The listing builds one solid part. Answer for the finished solid, in the listing's coordinates (mm). A direction names the side the tool comes from. Coordinates: 2 decimals unless noted, no trailing zeros. Loops run counter-clockwise (first coordinate to the right, second up) from the corner with the lowest first, then second, coordinate; pieces in that order, holes last. Notation, with made-up numbers: (68.5, -6.5) -> (89.5, -6.5) arc R25 cw to (89.5, 19.5) -> close; hole circle Ø1 at (70, -30.75). An arc over 180 degrees is marked (long way). Answer in a Markdown table with one row per item.
```python
from build123d import *

# Parameters (mm, degrees)
PAD003_DEPTH        = 1.6
SKETCH006_R         = 3.75
PAD004_DEPTH        = 3.6
HOLE001_D           = 3.6
HOLE001_DEPTH       = 25
HOLE001_CSINK_D     = 6.7
HOLE001_CSINK_ANGLE = 90


with BuildPart() as part:
    # Sketch005 → Pad003 (new body)
    with BuildSketch(Plane.XY):
        with BuildLine():
            Line((-49.75, 4.75), (49.75, 4.75))
            ThreePointArc((49.75, -4.75), (54.5, 0), (49.75, 4.75))
            Line((49.75, -4.75), (-49.75, -4.75))
            ThreePointArc((-49.75, 4.75), (-54.5, 0), (-49.75, -4.75))
        make_face()
    extrude(amount=PAD003_DEPTH)

    # Sketch006 → Pad004 (join)
    with BuildSketch(Plane.XY):
        with Locations((-49.75, 0)):
            Circle(SKETCH006_R)
        with Locations((-9.75, 0)):
            Circle(SKETCH006_R)
        with Locations((9.75, 0)):
            Circle(SKETCH006_R)
        with Locations((49.75, 0)):
            Circle(SKETCH006_R)
    extrude(amount=PAD004_DEPTH)

    # Hole001
    with Locations(Plane(origin=(0, 0, 0), x_dir=(1, 0, 0), z_dir=(0, 0, -1))):
        with Locations((-49.75, 0), (-9.75, 0), (9.75, 0), (49.75, 0)):
            CounterSinkHole(HOLE001_D / 2, HOLE001_CSINK_D / 2, depth=HOLE001_DEPTH, counter_sink_angle=HOLE001_CSINK_ANGLE)


with BuildPart() as part_1:
    # Body001 placement: moved
    add(part.part.moved(Location((0, 36, -32))))


solid = part_1.part
```
Item 1: A cutting plane is placed at C-C, the plane y = 36. Count the separate pieces of the cut face and the enclosed holes in it, plus the area to 3 significant figures.
Findings below:
| item | result |
|---|---|
| separate pieces | 5 |
| enclosed holes | 0 |
| area | 173 mm2 |
Item 2: A cutting plane is placed at A-A, the plane z = -29.75. Determine the outline of the cut face in (x, y), plus the area to 3 significant figures.
Findings below:
| item | result |
|---|---|
| outline | circle Ø7.5 at (-49.75, 36); circle Ø7.5 at (-9.75, 36); circle Ø7.5 at (9.75, 36); circle Ø7.5 at (49.75, 36); hole circle Ø3.6 at (-49.75, 36); hole circle Ø3.6 at (-9.75, 36); hole circle Ø3.6 at (9.75, 36); hole circle Ø3.6 at (49.75, 36) |
| area | 136 mm2 |
Item 3: Find the intervals of material crossed by probe 1 along Y at (x, z) = (-9.75, -29.65); probe 2 along X at (y, z) = (37.5, -30.55); probe 3 along X at (y, z) = (38.25, -30.2), in increasing order.
Findings below:
| item | result |
|---|---|
| probe 1 | y = 32.25 to 34.2, 37.8 to 39.75 |
| probe 2 | x = -54.26 to -50.92, -48.58 to -10.92, -8.58 to 8.58, 10.92 to 48.58, 50.92 to 54.26 |
| probe 3 | x = -52.75 to -46.75, -12.75 to -6.75, 6.75 to 12.75, 46.75 to 52.75 |
Item 4: Determine the mould class of faces 1 (the face through (-9.516, 34.215, -29.411)), 2 (the face through (-8, 37, -28.4)), 3 (the face through (-12.726, 33.718, -29.414)), 4 (the face through (-54.5, 36.1, -31.2)) for opening direction X: +X half, -X half, draft (parallel to the pull), parting line (faces both ways), or undercut.
Findings below:
| item | result |
|---|---|
| face 1 | undercut |
| face 2 | draft |
| face 3 | undercut |
| face 4 | -X half |
Item 5: A tool of negligible diameter and unlimited length cuts with its end or side. For faces 5 (the face through (-1, 36, -32)), 6 (the face through (46.774, 33.718, -29.414)), from which of +Z, -Z, +X, -X, +Y, -Y can it reach the whole face along a straight path? Write none if from no direction.
Findings below:
| item | result |
|---|---|
| face 5 | -Z, +X, -X, +Y, -Y |
| face 6 | +Z |
Item 6: A cutting plane is placed at B-B, the plane x = -9.75. Determine the outline of the cut face in (y, z).
Findings below:
| item | result |
|---|---|
| outline | (31.25, -32) -> (32.65, -32) -> (34.2, -30.45) -> (34.2, -28.4) -> (32.25, -28.4) -> (32.25, -30.4) -> (31.25, -30.4) -> close; (37.8, -30.45) -> (39.35, -32) -> (40.75, -32) -> (40.75, -30.4) -> (39.75, -30.4) -> (39.75, -28.4) -> (37.8, -28.4) -> close |
Item 7: Flat-ended cylindrical pins translate along their axes: pin 1 Ø3 at (x, y) = (1, 36) entering from +Z; pin 2 Ø1 at (y, z) = (39.5, -31) entering from -X; pin 3 Ø4 at (x, y) = (9.75, 36) entering from -Z. Find the tip coordinate at first contact, or state that the pin passes through.
Findings below:
| item | result |
|---|---|
| pin 1 | stops at z = -30.4 |
| pin 2 | stops at x = -53.43 |
| pin 3 | stops at z = -30.65 |
Item 8: A cutting plane is placed at D-D, the plane x = -33.5. Determine the outline of the cut face in (y, z), plus the area to 3 significant figures.
Findings below:
| item | result |
|---|---|
| outline | (31.25, -32) -> (40.75, -32) -> (40.75, -30.4) -> (31.25, -30.4) -> close |
| area | 15.2 mm2 |
